Geometry check sheet. Reference: the model listing, model coordinates, mm. Face numbers are marked on the shaded views. A direction names the side the tool comes from. Coordinates: 2 decimals unless noted, no trailing zeros. Order: outer loops, then holes, each group sorted by start corner. A loop starts at its lowest first (then second) coordinate and runs counter-clockwise, first axis right, second up. Notation, with made-up numbers: (4.25, 6.25) - (12.25, 6.25) arc R19 ccw to (12.25, 18.25) - close; hole circle Ø11 at (32, -3). An arc over 180 degrees is marked (long way). Put each result on its own line as item: value.
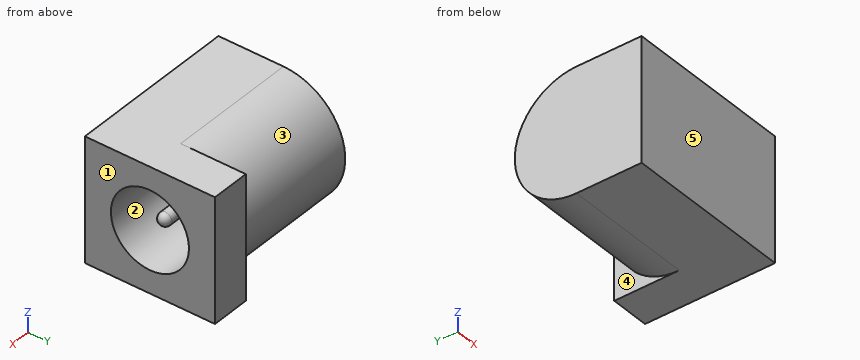
from build123d import *

# Parameters (mm, degrees)
BOSS_EXTRUDE1_DEPTH = 10
SKETCH2_W           = 9.5
SKETCH2_H           = 10
BOSS_EXTRUDE2_DEPTH = 3
SKETCH3_R           = 3
CUT_EXTRUDE1_DEPTH  = 12
SKETCH4_R           = 0.5
BOSS_EXTRUDE3_DEPTH = 11
FILLET1_R           = 0.5


with BuildPart() as part:
    # Sketch1 → Boss-Extrude1 (new body)
    with BuildSketch(Plane(origin=(0, 0, 0), x_dir=(0, 0, -1), z_dir=(1, 0, 0))):
        with BuildLine():
            Line((-4.75, -2.5), (4.75, -2.5))
            Line((4.75, -2.5), (4.75, 2.5))
            ThreePointArc((4.75, 2.5), (0, 7.25), (-4.75, 2.5))
            Line((-4.75, 2.5), (-4.75, -2.5))
        make_face()
    extrude(amount=BOSS_EXTRUDE1_DEPTH)

    # Sketch2 → Boss-Extrude2 (add)
    with BuildSketch(Plane(origin=(10, 0, 0), x_dir=(0, 0, -1), z_dir=(1, 0, 0))):
        with Locations((0, 2.5)):
            Rectangle(SKETCH2_W, SKETCH2_H)
    extrude(amount=BOSS_EXTRUDE2_DEPTH)

    # Sketch3 → Cut-Extrude1 (cut)
    with BuildSketch(Plane(origin=(13, 0, 0), x_dir=(0, 0, -1), z_dir=(1, 0, 0))):
        with Locations((0, 2.5)):
            Circle(SKETCH3_R)
    extrude(amount=-CUT_EXTRUDE1_DEPTH, mode=Mode.SUBTRACT)

    # Sketch4 → Boss-Extrude3 (add)
    with BuildSketch(Plane(origin=(1, 0, 0), x_dir=(0, 0, -1), z_dir=(1, 0, 0))):
        with Locations((0, 2.5)):
            Circle(SKETCH4_R)
    extrude(amount=BOSS_EXTRUDE3_DEPTH)

    # Fillet1
    fillet1_edges = [part.edges().sort_by_distance(p)[0] for p in [
        (12, 2.5, 0.5),
    ]]
    fillet(fillet1_edges, radius=FILLET1_R)


solid = part.part
Q1. Section check D-D on z = -1. Record the boundary of the cut face in (x, y), then the cut area to 3 significant figures.
Answer block:
outline: (0, -2.5) - (13, -2.5) - (13, -0.33) - (1, -0.33) - (1, 5.33) - (13, 5.33) - (13, 7.5) - (10, 7.5) - (10, 7.14) - (0, 7.14) - close
area: 58.6 mm^2
Q2. Section check A-A on x = 3.25. Record the boundary of the cut face in (y, z), then the cut area to 3 significant figures.
Answer block:
outline: (-2.5, -4.75) - (2.5, -4.75) arc R4.75 ccw to (2.5, 4.75) - (-2.5, 4.75) - close; circle Ø1 at (2.5, 0); hole circle Ø6 at (2.5, 0)
area: 55.5 mm^2
Q3. Section check B-B on z = 0. Record the boundary of the cut face in (x, y), then the cut area to 3 significant figures.
Answer block:
outline: (0, -2.5) - (13, -2.5) - (13, -0.5) - (1, -0.5) - (1, 2) - (11.5, 2) arc R0.5 ccw to (11.5, 3) - (1, 3) - (1, 5.5) - (13, 5.5) - (13, 7.5) - (10, 7.5) - (10, 7.25) - (0, 7.25) - close
area: 66.4 mm^2
Q4. Depth check by flat-ended pin: pin 1 Ø3 at (x, z) = (3.5, 0) entering from +Y. Enter the tip coordinate at first touch or a pass-through.
Answer block:
pin 1: stops at y = 7.25
Q5. Section check C-C on y = 1.75. Record the boundary of the cut face in (x, z).
Answer block:
outline: (0, -4.75) - (13, -4.75) - (13, -2.9) - (1, -2.9) - (1, 2.9) - (13, 2.9) - (13, 4.75) - (0, 4.75) - close
Q6. Thickness scan on L1, parallel to Y at x = 3.5, z = 0; L2, parallel to X at y = 3.5, z = -2; L3, parallel to Y at x = 12.75, z = 0.5. Record the ranges inside material, lowest first. Write a range as [from, to].
Answer block:
L1: y = [-2.5, -0.5], [2, 3], [5.5, 7.25]
L2: x = [0, 1]
L3: y = [-2.5, -0.46], [5.46, 7.5]
Q7. Access from +Z, -Z, +X, -X, +Y, -Y to the whole of each face (thin tool, end or side, straight path). Record for the marked faces 4 and 5.
Answer block:
face 4: -X, +Y
face 5: +Z, -Z, +X, -X, -Y
Q8. Draft check along Y on the marked faces 1, 2 and 3. Enter one of: pulls with the +Y half, pulls with the -Y half, needs draft (parallel to the pull), parting line crosses it, or undercut.
Answer block:
face 1: needs draft
face 2: undercut
face 3: pulls with the +Y half
